Answer from the drawing. Dimensions are ordinates in mm from the lowest x, y and z of the part. Round coordinates to 2 decimals unless told otherwise and drop trailing zeros. Loops run counter-clockwise (first coordinate to the right, second up) from the corner with the lowest first, then second, coordinate; pieces in that order, holes last. Notation, with made-up numbers: (7.5, 23) - (28.5, 23) arc R32 cw to (28.5, 59) - close; hole circle Ø10 at (41, 50.5). An arc over 180 degrees is marked (long way). Answer as CSV lines item,"result". Start each with the question number.
Q1. The mould has two halves that part along X. Classify the marked faces 1, 2, 3 and 4: +X half, -X half, draft (parallel to the pull), parting line (faces both ways), or undercut.
Q2. Each of these flat-tipped pins is pushed along its axis until it touches: pin 1 Ø1 at (x, y) = (7, 1.5) entering from +Z; pin 2 Ø4 at (y, z) = (3, 8) entering from +X. Where does it stop, or does it pass through?
Q3. Section C-C on y = 4 is taken. Write down the section's boundary in (x, z).
Q4. Straight lines are drawn through the part: L1, parallel to Z at x = 5, y = 6; L2, parallel to X at y = 5, z = 1; L3, parallel to X at y = 4.75, z = 6.5. For each, find the intervals that lie inside material, in ascending order. Write a range as [from, to].
Q5. Section B-B on z = 5 is taken. Write down the section's boundary in (x, y), then the cut area to 3 significant figures.
Q6. Section A-A on x = 5 is taken. Write down the section's boundary in (y, z), then the cut area to 3 significant figures.
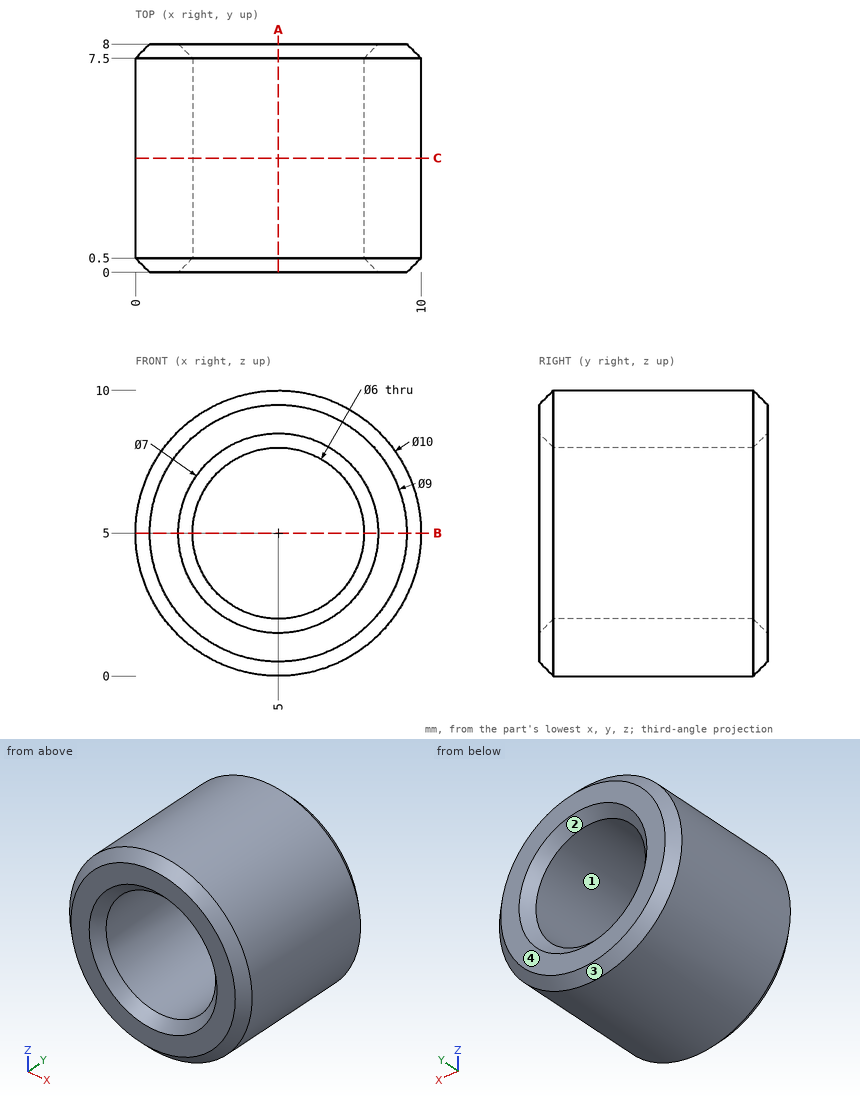
Findings:
1,face 1,"undercut"
1,face 2,"undercut"
1,face 3,"parting line"
1,face 4,"draft"
2,pin 1,"stops at z = 9.77"
2,pin 2,"stops at x = 9.9"
3,outline,"circle Ø10 at (5, 5); hole circle Ø6 at (5, 5)"
4,L1,"z = [0, 2], [8, 10]"
4,L2,"x = [2, 8]"
4,L3,"x = [0.23, 2.4], [7.6, 9.77]"
5,outline,"(0, 0.5) - (0.5, 0) - (1.5, 0) - (2, 0.5) - (2, 7.5) - (1.5, 8) - (0.5, 8) - (0, 7.5) - close; (8, 0.5) - (8.5, 0) - (9.5, 0) - (10, 0.5) - (10, 7.5) - (9.5, 8) - (8.5, 8) - (8, 7.5) - close"
5,area,"31.0 mm^2"
6,outline,"(0, 0.5) - (0.5, 0) - (7.5, 0) - (8, 0.5) - (8, 1.5) - (7.5, 2) - (0.5, 2) - (0, 1.5) - close; (0, 8.5) - (0.5, 8) - (7.5, 8) - (8, 8.5) - (8, 9.5) - (7.5, 10) - (0.5, 10) - (0, 9.5) - close"
6,area,"31.0 mm^2"
